Model file for the job. Use its own axes, mm. A direction names the side the tool comes from. Coordinates: 2 decimals unless noted, no trailing zeros. Order: outer loops, then holes, each group sorted by start corner. A loop starts at its lowest first (then second) coordinate and runs counter-clockwise, first axis right, second up.
Autodesk Inventor part; units mm, degrees
ref_plane "YZ Plane" through (0, 0, 0) normal (1, 0, 0) x (0, 1, 0)
ref_plane "XZ Plane" through (0, 0, 0) normal (0, 1, 0) x (-1, 0, 0)
ref_plane "XY Plane" through (0, 0, 0) normal (0, 0, 1) x (1, 0, 0)
sketch "Skizze5" plane through (0, 0, 0) normal (0, 0, 1) x (1, 0, 0)
  circle A0 centre (0, 0) radius 22
  line L0 (-30, 28.25) -> (30, 28.25)
  line L1 (30, 28.25) -> (30, -28.25)
  line L2 (30, -28.25) -> (-30, -28.25)
  line L3 (-30, -28.25) -> (-30, 28.25)
  dimension "d26" = 44
  dimension "d27" = 60
  dimension "d28" = 56.5
  dimension "d29" = 30
  dimension "d30" = 28.25
extrude "Extrusion2" add sketch "Skizze5" along normal blind 40
sketch "Skizze6" plane through (-30, 28.25, 0) normal (0, 1, 0) x (1, 0, 0)
  line L0 (60, -40) -> (0, -40)
  line L1 (60, 0) -> (60, -40)
  point P0 (30, 0)
  point P1 (30, -15)
  dimension "d34" = 30
  dimension "d73" = 15
hole "Bohrung3" at (0, 28.25, 15) direction (0, -1, 0) diameter 16.918 depth 41.1 tip angle 118
sketch "Skizze7" plane through (0, 0, 40) normal (0, 0, 1) x (1, 0, 0)
  circle A0 centre (0, 0) radius 25.5
  dimension "d42" = 51
extrude "Extrusion3" cut sketch "Skizze7" against normal blind 10
chamfer "Fase1" distance 0.5 angle 45 3 edges at (-25.5, 0, 40) (-22, 0, 30) (-22, 0, 0)
sketch "Skizze9" plane through (0, 0, 0) normal (0, 0, -1) x (-1, 0, 0)
  line L0 (30, 28.25) -> (-30, 28.25)
  line L1 (30, -28.25) -> (30, 28.25)
  point P0 (0, 0)
  point P1 (-24, -24)
  point P2 (-24, 22.25)
  point P3 (24, 22.25)
  point P4 (24, -24)
  dimension "d77" = 46.25
  dimension "d78" = 48
  dimension "d79" = 6
  dimension "d80" = 6
hole "Bohrung6" at (24, -24, 0) at (24, 22.25, 0) at (-24, 22.25, 0) at (-24, -24, 0) direction (0, 0, 1) diameter 4.134 depth 14.2 tip angle 118
sketch "Skizze10" plane through (-30, -28.25, 0) normal (0, -1, 0) x (1, 0, 0)
  line L0 (60, 0) -> (0, 0)
  line L1 (0, 40) -> (60, 40)
  line L2 (0, 0) -> (60, 0)
  line L3 (60, 0) -> (60, 40)
  line L4 (60, 40) -> (0, 40)
  line L5 (0, 40) -> (0, 0)
  point P0 (30, 0)
extrude "Extrusion4" add sketch "Skizze10" along normal blind 1.75
sketch "Skizze11" plane through (0, 0, 0) normal (0, 1, 0) x (-1, 0, 0)
  line L0 (-26.5, 36) -> (-25, 36)
  line L1 (-25, 36) -> (-25, 33)
  line L2 (-25, 33) -> (-26.5, 33)
  line L3 (-26.5, 33) -> (-26.5, 36)
  line L4 (0, -8) -> (0, 48)
  point P0 (0, 0)
  dimension "d90" = 1.5
  dimension "d91" = 25
  dimension "d92" = 33
  dimension "d93" = 3
revolve "Umdrehung1" cut sketch "Skizze11" angle 360 about axis through (0, 0, -10) along (0, 0, 1)
properties part number "Sensoraufnahme" material "Aluminium 6061"
Q1. Probe line 1 (X direction, y = -24, z = 6.75); line 2 (Y direction, x = -24, z = 11); line 3 (Y direction, x = 0, z = 32.2). List the from-to ranges inside material, lowest first.
Established:
line 1: x = -30 to -26.07, -21.93 to 21.93, 26.07 to 30
line 2: y = -30 to -26.07, -21.93 to 20.18, 24.32 to 28.25
line 3: y = -30 to -25.5, 25.5 to 28.25
Q2. Drop flat-ended pins along their axis: P1, Ø3.5, axis at x = -24, y = -24, coming from the -Z side; P2, Ø16, axis at x = 0, y = -12, coming from the +Z side (3 decimals); P3, Ø2.5, axis at x = 24, y = -24, coming from the -Z side. Give the stop position or say it passes through.
Established:
P1: stops at z = 14.39
P2: passes through
P3: stops at z = 14.69
Q3. Cut at B-B, the plane z = 34. List the corners of the cut face in (x, y).
Established:
outline: (-30, -30) - (30, -30) - (30, 28.25) - (-30, 28.25) - close; hole circle Ø53 at (0, 0)
Q4. Cut at A-A, the plane x = 0. Count the separate pieces of the cut face and the enclosed holes in it, plus the area to 3 significant figures.
Established:
separate pieces: 3
enclosed holes: 0
area: 388 mm2
Q5. Mould opens along X. For faces 1 (the face through (23.38, -22.03, 7.2)), 2 (the face through (14, 19, 0)), 3 (the face through (-14, 22, 36)), 4 (the face through (30, 0, 20)) say: pulls with the +X half, pulls with the -X half, needs draft (parallel to the pull), parting line crosses it, or undercut.
Established:
face 1: undercut
face 2: needs draft
face 3: undercut
face 4: pulls with the +X half
Q6. Cut at C-C, the plane z = 28. List the corners of the cut face in (x, y), plus the area to 3 significant figures.
Established:
outline: (-30, -30) - (30, -30) - (30, 28.25) - (-30, 28.25) - close; hole circle Ø44 at (0, 0)
area: 1,970 mm2
Q7. Which spindle directions (+Z, -Z, +X, -X, +Y, -Y) get a long thin tool onto all of the face, cutting with end or side? Do faces 5 (the face through (-14, 22, 33)), 6 (the face through (0, -30, 20)), 7 (the face through (23.38, 24.22, 7.2)), 8 (the face through (0, -23, 30)). Say none if no direction does.
Established:
face 5: none
face 6: +Z, -Z, +X, -X, -Y
face 7: -Z
face 8: +Z
